```python
from build123d import *

# Parameters (mm, degrees)
SKETCH_R          = 15
PAD_DEPTH         = 7
SKETCH001_R       = 3
PAD001_DEPTH      = 5
SKETCH002_R       = 15
SKETCH002_R_2     = 14
PAD002_DEPTH      = 8.2
SKETCH003_W       = 50
SKETCH003_H       = 45
PAD003_DEPTH      = 5
SKETCH004_W       = 50
SKETCH004_H       = 45
SKETCH004_W_2     = 48
SKETCH004_H_2     = 43
PAD004_DEPTH      = 10
SKETCH005_R       = 5
POCKET_DEPTH      = 5.001
POCKET_DEPTH_BACK = -10.001
SKETCH006_R       = 3
POCKET001_DEPTH   = 4


with BuildPart() as part:
    # Sketch → Pad (new body)
    with BuildSketch(Plane.XY):
        Circle(SKETCH_R)
    extrude(amount=PAD_DEPTH)

    # Sketch001 → Pad001 (join)
    with BuildSketch(Plane.XY):
        with BuildLine():
            add(Edge.make_bspline(
                [(-9.089263, 11.932531), (-7.840475, 19.926179), (0, 24.511142), (7.840475, 19.926179), (9.089263, 11.932531)],
                knots=[0, 0, 0, 0, 0.5, 1, 1, 1, 1], degree=3))
            Line((9.089263, 11.932531), (-9.089263, 11.932531))
        make_face()
        with Locations((0, 18.468813)):
            Circle(SKETCH001_R, mode=Mode.SUBTRACT)
    extrude(amount=PAD001_DEPTH)

    # Sketch002 → Pad002 (join)
    with BuildSketch(Plane.XY):
        Circle(SKETCH002_R)
        Circle(SKETCH002_R_2, mode=Mode.SUBTRACT)
    extrude(amount=PAD002_DEPTH)

    # Sketch003 → Pad003 (join)
    with BuildSketch(Plane.XY):
        with Locations((0, 2.5)):
            Rectangle(SKETCH003_W, SKETCH003_H)
    extrude(amount=-PAD003_DEPTH)

    # Sketch004 → Pad004 (join)
    with BuildSketch(Plane.XY):
        with Locations((0, 2.5)):
            Rectangle(SKETCH004_W, SKETCH004_H)
        with Locations((0, 2.5)):
            Rectangle(SKETCH004_W_2, SKETCH004_H_2, mode=Mode.SUBTRACT)
    extrude(amount=PAD004_DEPTH)

    # Sketch005 → Pocket (cut, two sides)
    with BuildSketch(Plane.XY) as pocket_sk:
        Circle(SKETCH005_R)
    extrude(amount=-POCKET_DEPTH, mode=Mode.SUBTRACT)
    extrude(pocket_sk.sketch, amount=-POCKET_DEPTH_BACK, mode=Mode.SUBTRACT)

    # Sketch006 → Pocket001 (cut)
    with BuildSketch(Plane.XY):
        with Locations((0, 18.468813)):
            Circle(SKETCH006_R)
    extrude(amount=-POCKET001_DEPTH, mode=Mode.SUBTRACT)


solid = part.part
```
The model under review builds one solid part; all positions refer to its coordinate system, in mm. A direction names the side the tool comes from. Give positions to 0.01 mm unless a question says otherwise; leave off trailing zeros. Loops run counter-clockwise (first coordinate to the right, second up) from the corner with the lowest first, then second, coordinate; pieces in that order, holes last. Notation, with made-up numbers: (63.5, 28.5) - (82.5, 28.5) arc R22 cw to (82.5, 61.5) - close; hole circle Ø5 at (-39, 57.25). An arc over 180 degrees is marked (long way). Answer as a JSON object with one key per item and string values.
Q1. Add section A-A on y = 0. State the section outline as (x, z) points, plus the area to 3 significant figures.
Worked out:
{"outline": "(-25, -5) - (-5, -5) - (-5, 7) - (-14, 7) - (-14, 8.2) - (-15, 8.2) - (-15, 0) - (-24, 0) - (-24, 10) - (-25, 10) - close; (5, -5) - (25, -5) - (25, 10) - (24, 10) - (24, 0) - (15, 0) - (15, 8.2) - (14, 8.2) - (14, 7) - (5, 7) - close", "area": "362 mm^2"}
Q2. Add section B-B on z = 6.25. State the section outline as (x, y) points, plus the area to 3 significant figures.
Worked out:
{"outline": "(-25, -20) - (25, -20) - (25, 25) - (-25, 25) - close; circle Ø30 at (0, 0); hole (-24, -19) - (24, -19) - (24, 24) - (-24, 24) - close; hole circle Ø10 at (0, 0)", "area": "814 mm^2"}
Q3. Mouldability with a two-part tool opening along Y and no side actions: class faces 1 (the flat face through (0, -20, 2)), 2 (the flat face through (25, 2, 2)), 3 (the flat face through (0, -6, 7)) as +Y half, -Y half, draft (parallel to the pull), parting line (faces both ways), or undercut.
Worked out:
{"face 1": "-Y half", "face 2": "draft", "face 3": "undercut"}
Q4. Add section D-D on z = -3.25. State the section outline as (x, y) points, plus the area to 3 significant figures.
Worked out:
{"outline": "(-25, -20) - (25, -20) - (25, 25) - (-25, 25) - close; hole circle Ø10 at (0, 0); hole circle Ø6 at (0, 18.47)", "area": "2,140 mm^2"}
Q5. Insertion check: pin 1 (9 mm diameter, centred on x = 0, y = 0, fed in from +Z); pin 2 (5 mm diameter, centred on x = 12, y = 13, fed in from +Z); pin 3 (6.5 mm diameter, centred on x = -1.5, y = 17, fed in from +Z); pin 4 (8.5 mm diameter, centred on x = -7, y = -3, fed in from +Z). Each pin has a flat end and moves straight along its axis. Give the tip position at first contact, or say it passes through.
Worked out:
{"pin 1": "passes through", "pin 2": "stops at z = 0", "pin 3": "stops at z = 8.2", "pin 4": "stops at z = 7"}
Q6. For faces 4 (the cylindrical face through (-0.391, 21.443, 0.437)), 5 (the cylindrical face through (-1.08, -4.88, 1.08)), list the 3-axis set-ups (+Z, -Z, +X, -X, +Y, -Y) from which the entire face can be reached by the end or side of a thin tool; tool diameter is ignored.
Worked out:
{"face 4": "+Z", "face 5": "+Z, -Z"}
Q7. Add section C-C on x = 18.5. State the section outline as (y, z) points, plus the area to 3 significant figures.
Worked out:
{"outline": "(-20, -5) - (25, -5) - (25, 10) - (24, 10) - (24, 0) - (-19, 0) - (-19, 10) - (-20, 10) - close", "area": "245 mm^2"}
Q8. To check wall thickness, follow line 1 along X through (y, z) = (0, 7.45); line 2 along Y through (x, z) = (0, -2); line 3 along X through (y, z) = (0, 0.75). State the ranges of each line that lie inside material, in increasing order.
Worked out:
{"line 1": "x = -25 to -24, -15 to -14, 14 to 15, 24 to 25", "line 2": "y = -20 to -5, 5 to 15.47, 21.47 to 25", "line 3": "x = -25 to -24, -15 to -5, 5 to 15, 24 to 25"}
